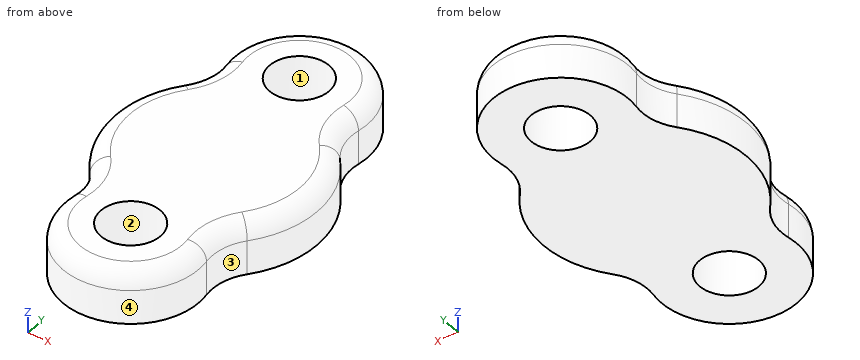
from build123d import *

# Parameters (mm, degrees)
SKETCH1_R           = 1.75
BOSS_EXTRUDE1_DEPTH = 3
FILLET1_R           = 1


with BuildPart() as part:
    # Sketch1 → Boss-Extrude1 (new body)
    with BuildSketch(Plane.XY):
        with BuildLine():
            ThreePointArc((-110.795927452, 3.007150415), (-112.200010897, -0.849992442), (-110.795927452, -4.707135299))
            ThreePointArc((-110.795927452, -4.707135299), (-110.196213999, -5.858855042), (-110.139367944, -7.156114891))
            ThreePointArc((-110.139367944, -7.156114891), (-106.200010897, -11.849992442), (-102.26065385, -7.156114891))
            ThreePointArc((-102.26065385, -7.156114891), (-102.203807795, -5.858855042), (-101.604094342, -4.707135299))
            ThreePointArc((-101.604094342, -4.707135299), (-100.200010897, -0.849992442), (-101.604094342, 3.007150415))
            ThreePointArc((-101.604094342, 3.007150415), (-102.203807795, 4.158870157), (-102.26065385, 5.456130007))
            ThreePointArc((-102.26065385, 5.456130007), (-106.200010897, 10.150007558), (-110.139367944, 5.456130007))
            ThreePointArc((-110.139367944, 5.456130007), (-110.196213999, 4.158870157), (-110.795927452, 3.007150415))
        make_face()
        with Locations((-106.200010897, 6.150007558)):
            Circle(SKETCH1_R, mode=Mode.SUBTRACT)
        with Locations((-106.200010897, -7.849992442)):
            Circle(SKETCH1_R, mode=Mode.SUBTRACT)
    extrude(amount=BOSS_EXTRUDE1_DEPTH)

    # Fillet1
    fillet1_edges = [part.edges().sort_by_distance(p)[0] for p in [
        (-102.203807795, -5.858855042, 3),
        (-100.200010897, -0.849992442, 3),
        (-102.203807795, 4.158870157, 3),
        (-106.200010897, 10.150007558, 3),
        (-110.196213999, 4.158870157, 3),
        (-112.200010897, -0.849992442, 3),
        (-110.196213999, -5.858855042, 3),
        (-106.200010897, -11.849992442, 3),
    ]]
    fillet(fillet1_edges, radius=FILLET1_R)


solid = part.part
CAD build for the part. Positions are in the model's coordinates, mm. Face numbers are marked on the shaded views. Coordinates: 2 decimals unless noted, no trailing zeros. Order: outer loops, then holes, each group sorted by start corner. A loop starts at its lowest first (then second) coordinate and runs counter-clockwise, first axis right, second up.
Item 1: Two-plate mould, pull along X, no slides. Class the marked faces 1, 2, 3 and 4: +X half, -X half, draft (parallel to the pull), parting line (faces both ways), or undercut.
Check sheet entries:
face 1: undercut
face 2: undercut
face 3: +X half
face 4: parting line
Item 2: Pin check, flat tips, straight feed: pin 1 Ø1 at (y, z) = (-7.5, 1) entering from +X; pin 2 Ø3 at (x, y) = (-106.2, -7.85) entering from -Z. Stop position of each tip, or through.
Check sheet entries:
pin 1: stops at x = -102.2
pin 2: passes through
Item 3: Band-saw the part on B-B on x = -105.25. Give the number of separate pieces and of enclosed holes in the cut face, plus the area to 3 significant figures.
Check sheet entries:
separate pieces: 3
enclosed holes: 0
area: 47.2 mm2
Item 4: Band-saw the part on A-A on z = 2.3. List the corners of the cut face in (x, y), plus the area to 3 significant figures.
Check sheet entries:
outline: (-110.76, -4.68) arc R3.05 cw to (-110.09, -7.16) arc R3.95 ccw (long way) to (-102.31, -7.16) arc R3.05 cw to (-101.64, -4.68) arc R5.95 ccw to (-101.64, 2.98) arc R3.05 cw to (-102.31, 5.46) arc R3.95 ccw (long way) to (-110.09, 5.46) arc R3.05 cw to (-110.76, 2.98) arc R5.95 ccw to start; hole circle Ø3.5 at (-106.2, -7.85); hole circle Ø3.5 at (-106.2, 6.15)
area: 165 mm2
Item 5: Drill centre lines: L1, parallel to Y at x = -106.25, z = 0.9; L2, parallel to Y at x = -104.75, z = 2.05; L3, parallel to X at y = 5.5, z = 0.8. Where is each one in solid material? Low to high.
Check sheet entries:
L1: y = -11.85 to -9.6, -6.1 to 4.4, 7.9 to 10.15
L2: y = -11.58 to -8.83, -6.87 to 5.17, 7.13 to 9.88
L3: x = -110.15 to -107.82, -104.58 to -102.25
